Source: three-view drawing plus pictorial views. Frame: mm from the lowest corner of the part. Give positions to 0.01 mm unless a question says otherwise; leave off trailing zeros. Write each loop counter-clockwise with the first axis right and the second up, starting at its lowest first coordinate (ties: lowest second). Pieces come first, ordered by that corner, then holes. Notation, with made-up numbers: M -9,50.25 L 7,50.25 A21 cw 7,54.25 Z; hole C 63,-36 d1. An arc over 180 degrees is marked long. Return JSON: item names as keys, results as strings.
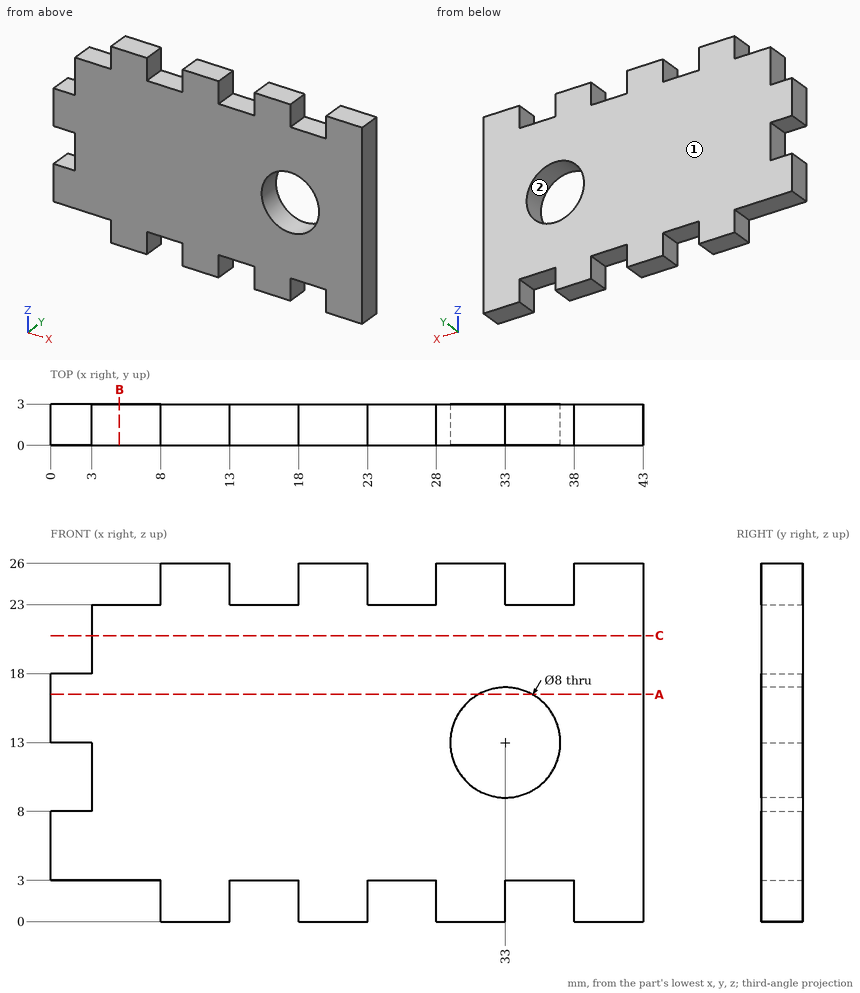
1) Cut plane C-C, the plane z = 20.75. Return the cut outline in (x, y), then the cut area to 3 significant figures.
Numbers:
{"outline": "M 3,0 L 43,0 L 43,3 L 3,3 Z", "area": "120 mm²"}
2) Cut plane B-B, the plane x = 5. Return the cut outline in (y, z).
Numbers:
{"outline": "M 0,3 L 3,3 L 3,23 L 0,23 Z"}
3) Draft query along Z for the marked faces 1 and 2. Return one class per face: released by +Z, released by -Z, zero draft, split by the parting line, or undercut.
Numbers:
{"face 1": "zero draft", "face 2": "undercut"}
4) Contact query for flat-ended pins moving along their axis: pin 1 Ø0.9 at (x, y) = (3, 1.5) entering from -Z; pin 2 Ø1.5 at (y, z) = (1, 24) entering from -X. Output: stop coordinate, or through.
Numbers:
{"pin 1": "stops at z = 3", "pin 2": "stops at x = 8"}
5) Cut plane A-A, the plane z = 16.5. Return the cut outline in (x, y).
Numbers:
{"outline": "M 0,0 L 31.06,0 L 31.06,3 L 0,3 Z; M 34.94,0 L 43,0 L 43,3 L 34.94,3 Z"}
6) Line query: line 1 (X direction, y = 1.45, z = 2.25); line 2 (Z direction, x = 26.5, y = 2.6); line 3 (X direction, y = 2.15, z = 15.25). Output: solid intervals per line, ascending. Write a range as [from, to].
Numbers:
{"line 1": "x = [8, 13], [18, 23], [28, 33], [38, 43]", "line 2": "z = [3, 23]", "line 3": "x = [0, 29.69], [36.31, 43]"}
